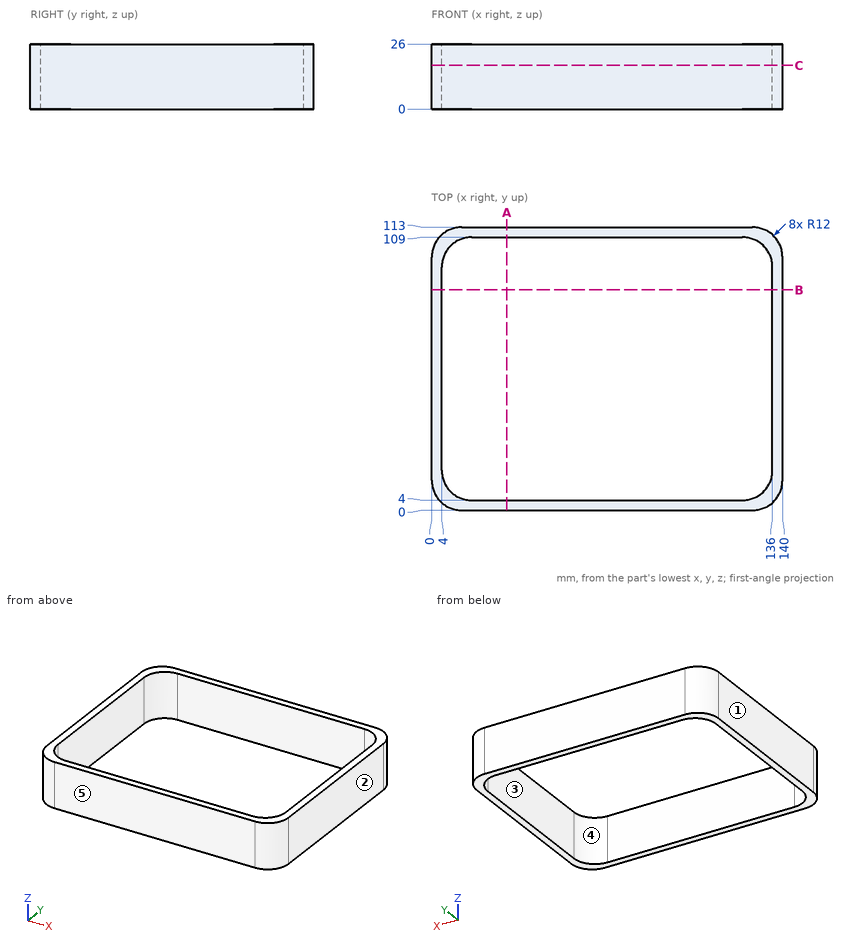
Input: dimensioned drawing with shaded views. Units: mm. Origin: part minimum x, y, z. A direction names the side the tool comes from. Give positions to 0.01 mm unless a question says otherwise; leave off trailing zeros. Order: outer loops, then holes, each group sorted by start corner. A loop starts at its lowest first (then second) coordinate and runs counter-clockwise, first axis right, second up. Notation, with made-up numbers: (22.25, -32) -> (69.25, -32) arc R36 ccw to (69.25, 7) -> close; hole circle Ø4 at (-13, 5). An arc over 180 degrees is marked (long way). Answer as a JSON object with one key per item and string values.
Q1. Section B-B (y = 88). Output: boundary loops of the cut face in (x, z).
Entries:
{"outline": "(0, 0) -> (4, 0) -> (4, 26) -> (0, 26) -> close; (136, 0) -> (140, 0) -> (140, 26) -> (136, 26) -> close"}
Q2. Draft query along X for the marked faces 1, 2 and 3. Return one class per face: released by +X, released by -X, zero draft, split by the parting line, or undercut.
Entries:
{"face 1": "released by -X", "face 2": "released by +X", "face 3": "undercut"}
Q3. Material intervals for probe 1 along Y at (x, z) = (90, 8.5); probe 2 along X at (y, z) = (67.5, 5.5); probe 3 along Y at (x, z) = (134, 5), sorted ascending.
Entries:
{"probe 1": "y = 0 to 4, 109 to 113", "probe 2": "x = 0 to 4, 136 to 140", "probe 3": "y = 1.61 to 9.37, 103.63 to 111.39"}
Q4. Section A-A (x = 30). Output: boundary loops of the cut face in (y, z), plus the area to 3 significant figures.
Entries:
{"outline": "(0, 0) -> (4, 0) -> (4, 26) -> (0, 26) -> close; (109, 0) -> (113, 0) -> (113, 26) -> (109, 26) -> close", "area": "208 mm^2"}
Q5. Access query for the marked faces 4 and 5. Directions: +Z, -Z, +X, -X, +Y, -Y. A direction counts if a zero-diameter tool reaches every point of the face in a straight line with its end or side. Return the directions, or none.
Entries:
{"face 4": "+Z, -Z", "face 5": "+Z, -Z, +X, -X, -Y"}
Q6. Section C-C (z = 17.5). Output: boundary loops of the cut face in (x, y).
Entries:
{"outline": "(0, 12) arc R12 ccw to (12, 0) -> (128, 0) arc R12 ccw to (140, 12) -> (140, 101) arc R12 ccw to (128, 113) -> (12, 113) arc R12 ccw to (0, 101) -> close; hole (4, 16) arc R12 ccw to (16, 4) -> (124, 4) arc R12 ccw to (136, 16) -> (136, 97) arc R12 ccw to (124, 109) -> (16, 109) arc R12 ccw to (4, 97) -> close"}
